Design review of the part built by this model. Coordinates are the model's own, in mm. A direction names the side the tool comes from. Give positions to 0.01 mm unless a question says otherwise; leave off trailing zeros. Loops run counter-clockwise (first coordinate to the right, second up) from the corner with the lowest first, then second, coordinate; pieces in that order, holes last.
from build123d import *

# Parameters (mm, degrees)
F5_DEPTH = 2
F3_R     = 1.875
F6_DEPTH = 10
F4_R     = 1.125
F7_DEPTH = 5


with BuildPart() as f5:
    # F2 (on Top) → F5 (new body)
    with BuildSketch(Plane.XY):
        with BuildLine():
            Line((-18, 22.242641), (-30.87868, 35.12132))
            ThreePointArc((-30.87868, 35.12132), (-35.12132, 35.12132), (-35.12132, 30.87868))
            Line((-35.12132, 30.87868), (-22.242641, 18))
            Line((-22.242641, 18), (-35.12132, 5.12132))
            ThreePointArc((-35.12132, 5.12132), (-35.12132, 0.87868), (-30.87868, 0.87868))
            Line((-30.87868, 0.87868), (-18, 13.757359))
            Line((-18, 13.757359), (-5.12132, 0.87868))
            ThreePointArc((-5.12132, 0.87868), (-0.87868, 0.87868), (-0.87868, 5.12132))
            Line((-0.87868, 5.12132), (-13.757359, 18))
            Line((-13.757359, 18), (-0.87868, 30.87868))
            ThreePointArc((-0.87868, 30.87868), (-0.87868, 35.12132), (-5.12132, 35.12132))
            Line((-5.12132, 35.12132), (-18, 22.242641))
        make_face()
    extrude(amount=F5_DEPTH)

    # F3 (on Top) → F6 (cut)
    with BuildSketch(Plane.XY):
        with Locations((-33, 33)):
            Circle(F3_R)
        with Locations((-3, 33)):
            Circle(F3_R)
        with Locations((-3, 3)):
            Circle(F3_R)
        with Locations((-33, 3)):
            Circle(F3_R)
    extrude(amount=F6_DEPTH, mode=Mode.SUBTRACT)

    # F4 (on Top) → F7 (join)
    with BuildSketch(Plane.XY):
        with Locations((-28, 8)):
            Circle(F4_R)
        with Locations((-8, 8)):
            Circle(F4_R)
        with Locations((-8, 28)):
            Circle(F4_R)
        with Locations((-28, 28)):
            Circle(F4_R)
    extrude(amount=F7_DEPTH)


solid = f5.part
Q1. Take a section at C-C (y = 8). Give the boundary of the cut face in (x, z) (3 decimals), plus the area to 3 significant figures.
Results:
outline: (-32.243, 0) - (-23.757, 0) - (-23.757, 2) - (-26.875, 2) - (-26.875, 5) - (-29.125, 5) - (-29.125, 2) - (-32.243, 2) - close; (-12.243, 0) - (-3.757, 0) - (-3.757, 2) - (-6.875, 2) - (-6.875, 5) - (-9.125, 5) - (-9.125, 2) - (-12.243, 2) - close
area: 47.4 mm2
Q2. Wall thickness on line 1 (Y direction, x = -33, z = 0.45) (3 decimals); line 2 (X direction, y = 3, z = 0.65) (3 decimals); line 3 (Z direction, x = -5, y = 8): over which ranges is each line inside the solid? List them lowest first.
Results:
line 1: y = 0 to 1.125, 4.875 to 7.243, 28.757 to 31.125, 34.875 to 36
line 2: x = -36 to -34.875, -31.125 to -28.757, -7.243 to -4.875, -1.125 to 0
line 3: z = 0 to 2
Q3. Insertion check: pin 1 (4 mm diameter, centred on x = -4, y = 12, fed in from +Z); pin 2 (1 mm diameter, centred on y = 9, z = 3.5, fed in from -X); pin 3 (5 mm diameter, centred on x = -3, y = 3, fed in from +Z); pin 4 (1 mm diameter, centred on x = -9.5, z = 1.5, fed in from -Y). Each pin has a flat end and moves straight along its axis. Give the tip position at first contact, or say it passes through.
Results:
pin 1: passes through
pin 2: stops at x = -29.01
pin 3: stops at z = 2
pin 4: stops at y = 4.76
Q4. Draft analysis for pull direction Y (two halves, no side actions). For faces 5 (the face through (-8, 8, 5)), 6 (the face through (-35.07, 35.17, 0.99)), 7 (the face through (-24.35, 28.59, 0.99)), state which applies: pulls with the +Y half, pulls with the -Y half, needs draft (parallel to the pull), parting line crosses it, or undercut.
Results:
face 5: needs draft
face 6: undercut
face 7: pulls with the +Y half
Q5. Take a section at D-D (x = -28). Give the boundary of the cut face in (y, z) (3 decimals), plus the area to 3 significant figures.
Results:
outline: (3.757, 0) - (12.243, 0) - (12.243, 2) - (9.125, 2) - (9.125, 5) - (6.875, 5) - (6.875, 2) - (3.757, 2) - close; (23.757, 0) - (32.243, 0) - (32.243, 2) - (29.125, 2) - (29.125, 5) - (26.875, 5) - (26.875, 2) - (23.757, 2) - close
area: 47.4 mm2
Q6. Take a section at A-A (z = 1.55). Give the boundary of the cut face in (x, y) (3 decimals).
Results:
outline: (-35.121, 5.121) arc R3 ccw to (-30.879, 0.879) - (-18, 13.757) - (-5.121, 0.879) arc R3 ccw to (-0.879, 5.121) - (-13.757, 18) - (-0.879, 30.879) arc R3 ccw to (-5.121, 35.121) - (-18, 22.243) - (-30.879, 35.121) arc R3 ccw to (-35.121, 30.879) - (-22.243, 18) - close; hole circle Ø3.75 at (-33, 3); hole circle Ø3.75 at (-33, 33); hole circle Ø3.75 at (-3, 3); hole circle Ø3.75 at (-3, 33)
Q7. Take a section at B-B (x = -3). Give the boundary of the cut face in (y, z) (3 decimals), plus the area to 3 significant figures.
Results:
outline: (0, 0) - (1.125, 0) - (1.125, 2) - (0, 2) - close; (4.875, 0) - (7.243, 0) - (7.243, 2) - (4.875, 2) - close; (28.757, 0) - (31.125, 0) - (31.125, 2) - (28.757, 2) - close; (34.875, 0) - (36, 0) - (36, 2) - (34.875, 2) - close
area: 14.0 mm2
Q8. Tool access review of faces 1 (the face through (-28.77, 24.53, 0.99)), 2 (the face through (-3.24, 34.86, 0.99)), 3 (the face through (-29.124, 28.049, 3.479)), 4 (the face through (-7.41, 24.35, 0.99)): name each direction out of +Z, -Z, +X, -X, +Y, -Y from which nothing blocks a thin tool from reaching the whole face with its end or side.
Results:
face 1: +Z, -Z, -X
face 2: +Z, -Z
face 3: +Z
face 4: +Z, -Z, +X
